Work out the finished part from the listing and answer in its coordinate system (mm). Round coordinates to 2 decimals unless told otherwise and drop trailing zeros. Write each loop counter-clockwise with the first axis right and the second up, starting at its lowest first coordinate (ties: lowest second). Pieces come first, ordered by that corner, then holes. Notation, with made-up numbers: (38.25, 35.25) - (57.25, 35.25) arc R32 cw to (57.25, 72.25) - close; hole circle Ø1 at (-33.5, 43). An arc over 180 degrees is marked (long way). Answer as a JSON object with one key per item and string values.
```python
from build123d import *

# Parameters (mm, degrees)
ESQUISSE1_R        = 1.5
BOSS_EXTRU_2_DEPTH = 3


with BuildPart() as part:
    # Esquisse1 → Boss.-Extru.2 (new body)
    with BuildSketch(Plane.XY):
        with BuildLine():
            ThreePointArc((-2.411034891, 11.820685714), (0, 10.75), (2.411034891, 11.820685714))
            ThreePointArc((2.411034891, 11.820685714), (3.975330286, 12.779130538), (5.80943088, 12.737759334))
            ThreePointArc((5.80943088, 12.737759334), (11.865562564, 7.430237213), (13.995977593, -0.335575935))
            ThreePointArc((13.995977593, -0.335575935), (13.382779595, -2.564868949), (11.442531564, -3.822325392))
            ThreePointArc((11.442531564, -3.822325392), (9.309773091, -5.375), (9.031496673, -7.998360322))
            ThreePointArc((9.031496673, -7.998360322), (9.079386541, -9.832302285), (8.126507731, -11.399994391))
            ThreePointArc((8.126507731, -11.399994391), (0.5019929, -13.990997217), (-7.288606081, -11.953084179))
            ThreePointArc((-7.288606081, -11.953084179), (-8.912631465, -10.307392628), (-9.031496673, -7.998360322))
            ThreePointArc((-9.031496673, -7.998360322), (-9.309773091, -5.375), (-11.442531564, -3.822325392))
            ThreePointArc((-11.442531564, -3.822325392), (-13.054716827, -2.946828253), (-13.935938611, -1.337764944))
            ThreePointArc((-13.935938611, -1.337764944), (-12.367555464, 6.560760004), (-6.707371512, 12.288660114))
            ThreePointArc((-6.707371512, 12.288660114), (-4.47014813, 12.872261577), (-2.411034891, 11.820685714))
        make_face()
        with Locations((9.309773091, 5.375)):
            Circle(ESQUISSE1_R, mode=Mode.SUBTRACT)
        with Locations((0, -10.75)):
            Circle(ESQUISSE1_R, mode=Mode.SUBTRACT)
        with Locations((-9.309773091, 5.375)):
            Circle(ESQUISSE1_R, mode=Mode.SUBTRACT)
        with Locations((5.375, -9.309773091)):
            Circle(ESQUISSE1_R, mode=Mode.SUBTRACT)
        with Locations((-5.375, 9.309773091)):
            Circle(ESQUISSE1_R, mode=Mode.SUBTRACT)
    extrude(amount=BOSS_EXTRU_2_DEPTH)


solid = part.part
```
Item 1: A cutting plane is placed at A-A (x = 0). Write down the section's boundary in (y, z), and give its area (4 significant figures).
Results found:
{"outline": "(-14, 0) - (-12.25, 0) - (-12.25, 3) - (-14, 3) - close; (-9.25, 0) - (10.75, 0) - (10.75, 3) - (-9.25, 3) - close", "area": "65.25 mm²"}
Item 2: A cutting plane is placed at B-B (z = 1.1). Give the number of separate pieces and of enclosed holes in the cut face, and give its area (3 significant figures).
Results found:
{"separate pieces": "1", "enclosed holes": "5", "area": "525 mm²"}
Item 3: A cutting plane is placed at D-D (y = 7.25). Write down the section's boundary in (x, z).
Results found:
{"outline": "(-11.98, 0) - (11.98, 0) - (11.98, 3) - (-11.98, 3) - close"}
Item 4: Each of these flat-tipped pins is pushed along its axis until it touches: P1, Ø2.5, axis at x = 0, y = -10.75, coming from the +Z side; P2, Ø1.5, axis at y = -7.5, z = 1, coming from the -X side. Where does it stop, or does it pass through?
Results found:
{"P1": "through", "P2": "x = -9.1"}
Item 5: A cutting plane is placed at C-C (x = -5.75). Write down the section's boundary in (y, z).
Results found:
{"outline": "(-12.76, 0) - (7.86, 0) - (7.86, 3) - (-12.76, 3) - close; (10.76, 0) - (12.76, 0) - (12.76, 3) - (10.76, 3) - close"}
Item 6: Consider line 1 along X through (y, z) = (6.5, 2.5); line 2 along X through (y, z) = (-11.5, 1.95); line 3 along Y through (x, z) = (-5.5, 1.3) (3 decimals). Determine where each line is inside the solid, lowest interval first.
Results found:
{"line 1": "-12.4 to -10.3, -8.32 to 8.32, 10.3 to 12.4", "line 2": "-8.01 to -1.3, 1.3 to 7.98", "line 3": "-12.874 to 7.815, 10.805 to 12.82"}
Item 7: Determine the mould class of faces 1 (the cylindrical face through (-0.325, -12.214, 1.479)), 2 (the flat face through (0, 0, 3)), 3 (the cylindrical face through (11.804, 7.527, 1.479)) for opening direction X: pulls with the +X half, pulls with the -X half, needs draft (parallel to the pull), parting line crosses it, or undercut.
Results found:
{"face 1": "undercut", "face 2": "needs draft", "face 3": "pulls with the +X half"}
